Design review of the part built by this model. Coordinates are the model's own, in mm. Give positions to 0.01 mm unless a question says otherwise; leave off trailing zeros. Order: outer loops, then holes, each group sorted by start corner. A loop starts at its lowest first (then second) coordinate and runs counter-clockwise, first axis right, second up.
```python
from build123d import *

# Parameters (mm, degrees)
PAD_DEPTH = 6


with BuildPart() as part:
    # Sketch → Pad (new body)
    with BuildSketch(Plane.XZ):
        with BuildLine():
            Line((0, 0), (215, 0))
            Line((215, 0), (215, 100))
            Line((215, 100), (167.5, 100))
            ThreePointArc((47.5, 100), (107.5, 10), (167.5, 100))
            Line((47.5, 100), (0, 100))
            Line((0, 100), (0, 0))
        make_face()
    extrude(amount=PAD_DEPTH)


solid = part.part
```
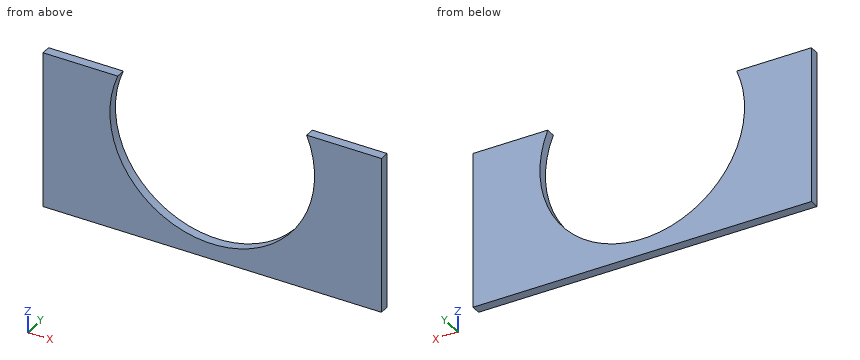
1. Take a section at A-A (z = 75). State the section outline as (x, y) points, then the cut area to 3 significant figures.
Recorded:
outline: (0, -6) - (42.5, -6) - (42.5, 0) - (0, 0) - close; (172.5, -6) - (215, -6) - (215, 0) - (172.5, 0) - close
area: 510 mm2
2. Take a section at D-D (z = 15.5). State the section outline as (x, y) points, then the cut area to 3 significant figures.
Recorded:
outline: (0, -6) - (81.33, -6) - (81.33, 0) - (0, 0) - close; (133.67, -6) - (215, -6) - (215, 0) - (133.67, 0) - close
area: 976 mm2
3. Take a section at B-B (y = -2.15). State the section outline as (x, z) points.
Recorded:
outline: (0, 0) - (215, 0) - (215, 100) - (167.5, 100) arc R65 cw (long way) to (47.5, 100) - (0, 100) - close
4. Take a section at C-C (x = 107.5). State the section outline as (y, z) points, then the cut area to 3 significant figures.
Recorded:
outline: (-6, 0) - (0, 0) - (0, 10) - (-6, 10) - close
area: 60.0 mm2
5. For line 1 along X through (y, z) = (-3.3, 75); line 2 along X through (y, z) = (-0.7, 54); line 3 along Z through (x, y) = (126, -5.5), list the stretches that pass through material, from the lowest coordinate up.
Recorded:
line 1: x = 0 to 42.5, 172.5 to 215
line 2: x = 0 to 45.99, 169.01 to 215
line 3: z = 0 to 12.69
6. For pin 1 (3 mm diameter, centred on y = -5, z = 74, fed in from -X), flat-tipped, find the tip position at first contact; note if it passes through.
Recorded:
pin 1: stops at x = 0
